Source: CAD feature listing. Evaluate the final solid. Frame: model axes, mm. A direction names the side the tool comes from. Round coordinates to 2 decimals unless told otherwise and drop trailing zeros. Order: outer loops, then holes, each group sorted by start corner. A loop starts at its lowest first (then second) coordinate and runs counter-clockwise, first axis right, second up. Notation, with made-up numbers: (-10.75, 38) - (18.25, 38) arc R11 cw to (18.25, 54) - close; hole circle Ø8 at (14, 5). An arc over 180 degrees is marked (long way). Put each result on its own line as item: value. Start each with the question number.
1) Line query: probe 1 along Y at (x, z) = (-17, 35); probe 2 along Z at (x, y) = (0, -22.5); probe 3 along X at (y, z) = (18, 27). Output: solid intervals per line, ascending. Write a range as [from, to].
2) Access query for faces 4 (the face through (24, 15, 40)), 5 (the face through (12.89, 13.11, 32.9)). Directions: +Z, -Z, +X, -X, +Y, -Y. A direction counts if a zero-diameter tool reaches every point of the face in a straight line with its end or side. Return the directions, or none.
3) Section C-C on x = 0. Output: boundary loops of the cut face in (y, z), then the cut area to 3 significant figures.
4) Mould query, pull axis Y, two halves, no side actions, for faces 1 (the face through (-1, 0, 0)), 2 (the face through (-16.501, 18, 37)), 3 (the face through (0, -15, 20)). Classes: +Y half, -Y half, draft (parallel to the pull), parting line (faces both ways), or undercut.
5) Section A-A on y = -21. Output: boundary loops of the cut face in (x, z), then the cut area to 3 significant figures.
6) Section B-B on z = 20. Output: boundary loops of the cut face in (x, y), then the cut area to 3 significant figures.
7) Contact query for a flat-ended pin moving along its axis: P1, Ø5, axis at x = 0.5, z = 20.5, coming from the -Y side. Output: stop coordinate, or through.
```python
from build123d import *

# Parameters (mm, degrees)
SKETCH1_W           = 75
SKETCH1_H           = 50
BOSS_EXTRUDE1_DEPTH = 40
SKETCH2_R           = 9.272983733
CUT_EXTRUDE1_DEPTH  = 14
SKETCH3_R           = 8.895673095
SKETCH3_R_2         = 2.676649409
BOSS_EXTRUDE2_DEPTH = 14
SKETCH4_R           = 2.552861956
BOSS_EXTRUDE3_DEPTH = 14
SKETCH5_W           = 18
SKETCH5_H           = 10
SKETCH5_W_2         = 17.211665491
SKETCH5_H_2         = 9.562036384
CUT_EXTRUDE2_DEPTH  = 7
SKETCH6_R           = 5
CUT_EXTRUDE3_DEPTH  = 10


with BuildPart() as part:
    # Sketch1 → Boss-Extrude1 (new body)
    with BuildSketch(Plane.XY):
        Rectangle(SKETCH1_W, SKETCH1_H)
    extrude(amount=BOSS_EXTRUDE1_DEPTH)

    # Sketch2 → Cut-Extrude1 (cut)
    with BuildSketch(Plane.XY.offset(40)):
        with Locations((21.778192922, 12.714084695)):
            Circle(SKETCH2_R)
    extrude(amount=-CUT_EXTRUDE1_DEPTH, mode=Mode.SUBTRACT)

    # Sketch3 → Boss-Extrude2 (add)
    with BuildSketch(Plane.XY.offset(26)):
        with Locations((21.778192922, 12.714084695)):
            Circle(SKETCH3_R)
        with Locations((21.778192922, 12.714084695)):
            Circle(SKETCH3_R_2, mode=Mode.SUBTRACT)
    extrude(amount=BOSS_EXTRUDE2_DEPTH)

    # Sketch4 → Boss-Extrude3 (add)
    with BuildSketch(Plane.XY.offset(26)):
        with Locations((21.778192922, 12.714084695)):
            Circle(SKETCH4_R)
    extrude(amount=BOSS_EXTRUDE3_DEPTH)

    # Sketch5 → Cut-Extrude2 (cut)
    with BuildSketch(Plane.XY.offset(40)):
        with Locations((-25.106926905, 17.674362133)):
            Rectangle(SKETCH5_W, SKETCH5_H)
        with Locations((-25.106926904, 17.674362133)):
            Rectangle(SKETCH5_W_2, SKETCH5_H_2, mode=Mode.SUBTRACT)
    extrude(amount=-CUT_EXTRUDE2_DEPTH, mode=Mode.SUBTRACT)

    # Sketch6 → Cut-Extrude3 (cut)
    with BuildSketch(Plane.XZ.offset(25)):
        with Locations((0, 20)):
            Circle(SKETCH6_R)
    extrude(amount=-CUT_EXTRUDE3_DEPTH, mode=Mode.SUBTRACT)


solid = part.part
```
Answer sheet:
1. probe 1: [-25, 12.67], [12.89, 22.46], [22.67, 25]
1. probe 2: [0, 15], [25, 40]
1. probe 3: [-37.5, 14.16], [14.62, 28.93], [29.4, 37.5]
2. face 4: +Z, +X, -X, +Y, -Y
2. face 5: +Z
3. outline: (-25, 0) - (25, 0) - (25, 40) - (-25, 40) - (-25, 25) - (-15, 25) - (-15, 15) - (-25, 15) - close
3. area: 1,900 mm^2
4. face 1: draft
4. face 2: undercut
4. face 3: -Y half
5. outline: (-37.5, 0) - (37.5, 0) - (37.5, 40) - (-37.5, 40) - close; hole circle Ø10 at (0, 20)
5. area: 2,920 mm^2
6. outline: (-37.5, -25) - (-5, -25) - (-5, -15) - (5, -15) - (5, -25) - (37.5, -25) - (37.5, 25) - (-37.5, 25) - close
6. area: 3,650 mm^2
7. P1: y = -15
